Check sheet for the drawn part. Datum: minimum x, y, z corner. Units: mm. A direction names the side the tool comes from. Round coordinates to 2 decimals unless told otherwise and drop trailing zeros. Loops run counter-clockwise (first coordinate to the right, second up) from the corner with the lowest first, then second, coordinate; pieces in that order, holes last. Notation, with made-up numbers: (-1, 66) -> (3, 66) arc R26 cw to (3, 92) -> close; hole circle Ø10 at (39, 80.25). An arc over 180 degrees is marked (long way). Write item = value, one per line. Start each with the question number.
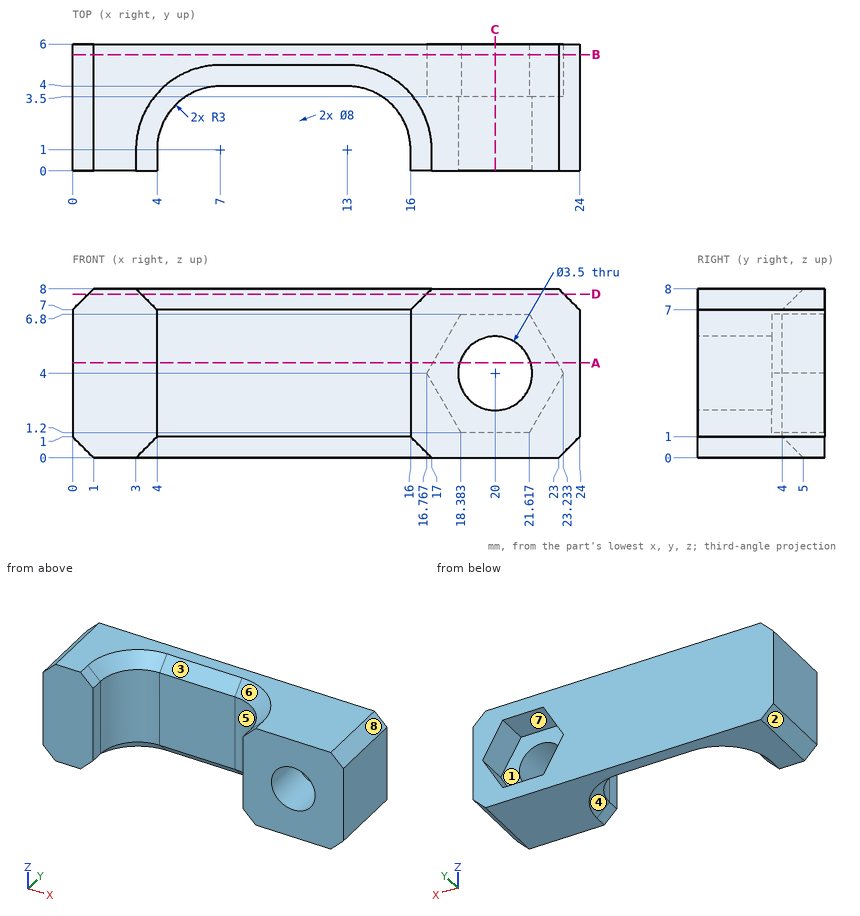
(1) Depth check by flat-ended pin: pin 1 Ø3 at (x, z) = (20.5, 3) entering from +Y; pin 2 Ø0.5 at (y, z) = (0.5, 5) entering from -X. Enter the tip coordinate at first touch or a pass-through.
(2) Section check A-A on z = 4.5. Enter the section's corners in (x, y) (1 decimal).
(3) Access from +Z, -Z, +X, -X, +Y, -Y to the whole of each face (thin tool, end or side, straight path). Record for the marked faces 4, 5, 6, 7 and 8.
(4) Section check D-D on z = 7.75. Enter the section's corners in (x, y).
(5) Section check C-C on x = 20. Enter the section's corners in (y, z).
(6) Scan lines: line 1 (Z direction, x = 20, y = 1.5); line 2 (X direction, y = 0.5, z = 6.5); line 3 (Z direction, x = 20.5, y = 5.5). Record each from-to range of solid material in increasing order. Write a range as [from, to].
(7) Section check B-B on y = 5.5. Enter the section's corners in (x, z), then the cut area to 3 significant figures.
(8) Draft check along Z on the marked faces 1, 2 and 3. Enter one of: +Z half, -Z half, draft (parallel to the pull), parting line (faces both ways), or undercut.
Computed values:
q1.pin_1 = 3.5
q1.pin_2 = 0
q2.outline = (0, 0) -> (4, 0) -> (4, 1) arc R3 cw to (7, 4) -> (13, 4) arc R3 cw to (16, 1) -> (16, 0) -> (18.3, 0) -> (18.3, 3.5) -> (17.1, 3.5) -> (17.1, 6) -> (0, 6) -> close; (21.7, 0) -> (24, 0) -> (24, 6) -> (22.9, 6) -> (22.9, 3.5) -> (21.7, 3.5) -> close
q3.face_4 = -Z, -Y
q3.face_5 = +Z, -Z, -Y
q3.face_6 = +Z, -Y
q3.face_7 = +Y
q3.face_8 = +Z, +X, +Y, -Y
q4.outline = (0.75, 0) -> (3.25, 0) -> (3.25, 1) arc R3.75 cw to (7, 4.75) -> (13, 4.75) arc R3.75 cw to (16.75, 1) -> (16.75, 0) -> (23.25, 0) -> (23.25, 6) -> (0.75, 6) -> close
q5.outline = (0, 0) -> (6, 0) -> (6, 1.2) -> (3.5, 1.2) -> (3.5, 2.25) -> (0, 2.25) -> close; (0, 5.75) -> (3.5, 5.75) -> (3.5, 6.8) -> (6, 6.8) -> (6, 8) -> (0, 8) -> close
q6.line_1 = [0, 2.25], [5.75, 8]
q6.line_2 = [0, 4], [16, 24]
q6.line_3 = [0, 1.2], [6.8, 8]
q7.outline = (0, 1) -> (1, 0) -> (23, 0) -> (24, 1) -> (24, 7) -> (23, 8) -> (1, 8) -> (0, 7) -> close; hole (16.77, 4) -> (18.38, 1.2) -> (21.62, 1.2) -> (23.23, 4) -> (21.62, 6.8) -> (18.38, 6.8) -> close
q7.area = 163 mm²
q8.face_1 = undercut
q8.face_2 = -Z half
q8.face_3 = +Z half
